Here's the drawing with two shaded views (mm, measured from the low corner). I have some questions. Round coordinates to 2 decimals unless told otherwise and drop trailing zeros. Order: outer loops, then holes, each group sorted by start corner. A loop starts at its lowest first (then second) coordinate and runs counter-clockwise, first axis right, second up.
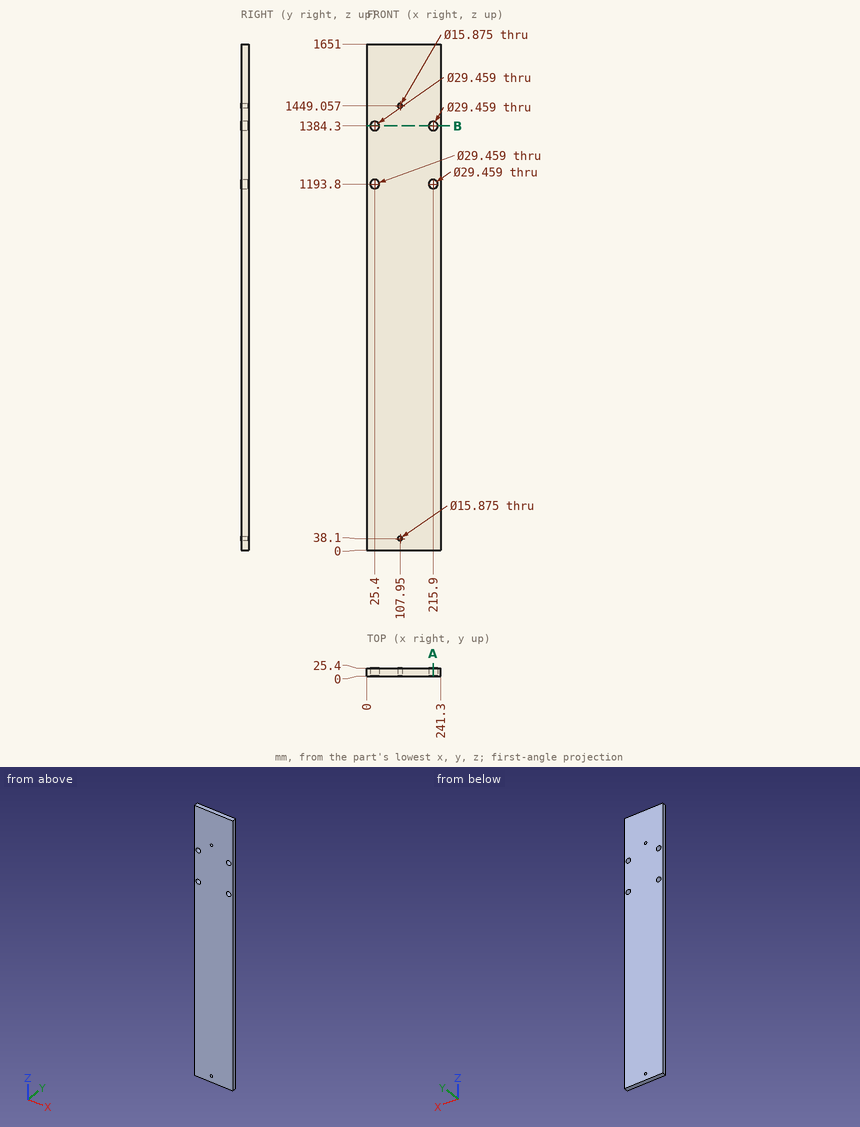
Q1. Imagine slicing it at A-A, the plane x = 215.9. Please give me the cut outline in (y, z), then the cut area to 3 significant figures.
Q2. I need wall thicknesses on L1, parallel to Z at x = 107.95, y = 19.75 (1 decimal); L2, parallel to X at y = 10.5, z = 1384.3; L3, parallel to Z at x = 15.5, y = 19.75 (1 decimal). Which ranges of each line are inside material? Lowest first, please.
Q3. Imagine slicing it at B-B, the plane z = 1384.3. Please give me the cut outline in (x, y), then the cut area to 3 significant figures.
Filled in:
1. outline: (0, 0) - (25.4, 0) - (25.4, 1179.07) - (0, 1179.07) - close; (0, 1208.53) - (25.4, 1208.53) - (25.4, 1369.57) - (0, 1369.57) - close; (0, 1399.03) - (25.4, 1399.03) - (25.4, 1651) - (0, 1651) - close
1. area: 40,400 mm2
2. L1: z = 0 to 30.2, 46 to 1441.1, 1457 to 1651
2. L2: x = 0 to 10.67, 40.13 to 201.17, 230.63 to 241.3
2. L3: z = 0 to 1182.9, 1204.7 to 1373.4, 1395.2 to 1651
3. outline: (0, 0) - (10.67, 0) - (10.67, 25.4) - (0, 25.4) - close; (40.13, 0) - (201.17, 0) - (201.17, 25.4) - (40.13, 25.4) - close; (230.63, 0) - (241.3, 0) - (241.3, 25.4) - (230.63, 25.4) - close
3. area: 4,630 mm2
